from build123d import *

# Parameters (mm, degrees)
BOSS_EXTRU_2_DEPTH      = 50
ESQUISSE5_R             = 1.75
ENL_V_MAT_EXTRU_2_DEPTH = 117.711988712
ESQUISSE6_R             = 1.75
ENL_V_MAT_EXTRU_3_DEPTH = 117.711988712
ENL_V_MAT_EXTRU_5_DEPTH = 44
ESQUISSE8_R             = 5
BOSS_EXTRU_3_DEPTH      = 100
ENL_V_MAT_EXTRU_6_DEPTH = 124.636564171
CONG_1_R                = 2.5
R_VOLUTION1_ANGLE       = 180
BOSS_EXTRU_4_DEPTH      = 1
CONG_2_R                = 10


with BuildPart() as part:
    # Esquisse4 → Boss.-Extru.2 (new body)
    with BuildSketch(Plane.XY):
        Polygon((-14.142135624, 45), (14.142135624, 45), (45, 14.142135624), (45, -14.142135624), (14.142135624, -45), (-14.142135624, -45), (-45, -14.142135624), (-45, 14.142135624), align=None)
    extrude(amount=BOSS_EXTRU_2_DEPTH)

    # Esquisse5 → Enlèv. mat.-Extru.2 (cut, through all)
    with BuildSketch(Plane(origin=(29.571067812, 29.571067812, 0), x_dir=(0, 0, -1), z_dir=(0.7071067811865474, 0.7071067811865477, 0))):
        with Locations(Location((-13.335, 11.665, 0), (0, 0, 90))):
            Circle(ESQUISSE5_R)
        with Locations(Location((-36.665, 11.665, 0), (0, 0, 90))):
            Circle(ESQUISSE5_R)
        with Locations(Location((-13.335, -11.665, 0), (0, 0, 90))):
            Circle(ESQUISSE5_R)
        with Locations(Location((-36.665, -11.665, 0), (0, 0, 90))):
            Circle(ESQUISSE5_R)
    extrude(amount=-ENL_V_MAT_EXTRU_2_DEPTH, mode=Mode.SUBTRACT)

    # Esquisse6 → Enlèv. mat.-Extru.3 (cut, through all)
    with BuildSketch(Plane(origin=(29.571067812, -29.571067812, 0), x_dir=(0, 0, -1), z_dir=(0.7071067811865476, -0.7071067811865476, 0))):
        with Locations(Location((-13.335, 11.665, 0), (0, 0, 90))):
            Circle(ESQUISSE6_R)
        with Locations((-36.665, 11.665)):
            Circle(ESQUISSE6_R)
        with Locations((-13.335, -11.665)):
            Circle(ESQUISSE6_R)
        with Locations((-36.665, -11.665)):
            Circle(ESQUISSE6_R)
    extrude(amount=-ENL_V_MAT_EXTRU_3_DEPTH, mode=Mode.SUBTRACT)

    # Esquisse7 → Enlèv. mat.-Extru.5 (cut)
    with BuildSketch(Plane.XY.offset(50)):
        Polygon((-40, 12.071067812), (-12.071067812, 40), (12.071067812, 40), (40, 12.071067812), (40, -12.071067812), (12.071067812, -40), (-12.071067812, -40), (-40, -12.071067812), align=None)
    extrude(amount=-ENL_V_MAT_EXTRU_5_DEPTH, mode=Mode.SUBTRACT)

    # Esquisse8 → Boss.-Extru.3 (add)
    with BuildSketch(Plane(origin=(0, 0, 0), x_dir=(-1, 0, 0), z_dir=(0, 0, -1))):
        Circle(ESQUISSE8_R)
    extrude(amount=BOSS_EXTRU_3_DEPTH)

    # Esquisse9 → Enlèv. mat.-Extru.6 (cut, through all)
    with BuildSketch(Plane.XY.offset(6)):
        Polygon((-13.017766953, 13.017766953), (-0.289844892, 25.745689014), (-9.128679656, 34.584523779), (-34.584523779, 9.128679656), (-25.745689014, 0.289844892), align=None)
        Polygon((25.745689014, -0.289844892), (34.584523779, -9.128679656), (9.128679656, -34.584523779), (0.289844892, -25.745689014), (13.017766953, -13.017766953), align=None)
        Polygon((-13.017766953, -13.017766953), (-23.624368671, -2.411165235), (-32.463203436, -11.25), (-11.25, -32.463203436), (-2.411165235, -23.624368671), align=None)
        Polygon((2.411165235, 23.624368671), (11.25, 32.463203436), (32.463203436, 11.25), (23.624368671, 2.411165235), (13.017766953, 13.017766953), align=None)
    extrude(amount=-ENL_V_MAT_EXTRU_6_DEPTH, mode=Mode.SUBTRACT)

    # Congé1
    cong_1_edges = [part.edges().sort_by_distance(p)[0] for p in [
        (2.411165235, 23.624368671, 3),
        (11.25, 32.463203436, 3),
        (32.463203436, 11.25, 3),
        (23.624368671, 2.411165235, 3),
        (-2.411165235, -23.624368671, 3),
        (-11.25, -32.463203436, 3),
        (-32.463203436, -11.25, 3),
        (-23.624368671, -2.411165235, 3),
        (25.745689014, -0.289844892, 3),
        (34.584523779, -9.128679656, 3),
        (9.128679656, -34.584523779, 3),
        (0.289844892, -25.745689014, 3),
        (-25.745689014, 0.289844892, 3),
        (-34.584523779, 9.128679656, 3),
        (-9.128679656, 34.584523779, 3),
        (-0.289844892, 25.745689014, 3),
    ]]
    fillet(cong_1_edges, radius=CONG_1_R)

    # Esquisse12 → Révolution1 (revolve)
    with BuildSketch(Plane(origin=(0, 0, -100), x_dir=(-1, 0, 0), z_dir=(0, 0, -1))):
        with BuildLine():
            Line((-5, 0), (5, 0))
            ThreePointArc((5, 0), (0, 5), (-5, 0))
        make_face()
    revolve(axis=Axis((5, 0, -100), (-1, 0, 0)), revolution_arc=R_VOLUTION1_ANGLE)

    # Esquisse13 → Boss.-Extru.4 (add)
    with BuildSketch(Plane.XY.offset(50)):
        Polygon((-45, 14.142135624), (-14.142135624, 45), (14.142135624, 45), (45, 14.142135624), (45, -14.142135624), (14.142135624, -45), (-14.142135624, -45), (-45, -14.142135624), align=None)
        Polygon((-40, 12.071067812), (-12.071067812, 40), (12.071067812, 40), (40, 12.071067812), (40, -12.071067812), (12.071067812, -40), (-12.071067812, -40), (-40, -12.071067812), align=None, mode=Mode.SUBTRACT)
    extrude(amount=BOSS_EXTRU_4_DEPTH)

    # Congé2
    cong_2_edges = [part.edges().sort_by_distance(p)[0] for p in [
        (5, 0, 0),
    ]]
    fillet(cong_2_edges, radius=CONG_2_R)


solid = part.part
Verification items for the finished model (mm, model axes). A direction names the side the tool comes from. Coordinates: 2 decimals unless noted, no trailing zeros. Order: outer loops, then holes, each group sorted by start corner. A loop starts at its lowest first (then second) coordinate and runs counter-clockwise, first axis right, second up.
Item 1: Material ranges on L1, parallel to Y at x = -5.5, z = 23.5; L2, parallel to Z at x = -37, y = -1, recorded low to high.
Filled in:
L1: y = -45 to -40, 40 to 45
L2: z = 0 to 6
Item 2: Section check A-A, the plane z = 20.5. Enter the section's corners in (x, y).
Filled in:
outline: (-45, -14.14) - (-14.14, -45) - (14.14, -45) - (45, -14.14) - (45, 14.14) - (14.14, 45) - (-14.14, 45) - (-45, 14.14) - close; hole (-40, -12.07) - (-12.07, -40) - (12.07, -40) - (40, -12.07) - (40, 12.07) - (12.07, 40) - (-12.07, 40) - (-40, 12.07) - close
Item 3: Release check for a two-part mould opening along X. For faces 1 (the face through (6.793, 28.007, 3.042)), 2 (the face through (-45, 0, 25)), 3 (the face through (29.787, -29.355, 25.143)), 4 (the face through (31.428, 11.277, 2.958)) record: +X half, -X half, draft (parallel to the pull), parting line (faces both ways), or undercut.
Filled in:
face 1: undercut
face 2: -X half
face 3: +X half
face 4: undercut
Item 4: Depth check by flat-ended pin: pin 1 (1.5 mm diameter, centred on x = 16.5, z = 10.5, fed in from +Y); pin 2 (3 mm diameter, centred on y = 20, z = 30.5, fed in from -X); pin 3 (3 mm diameter, centred on y = -23.5, z = 16, fed in from -X); pin 4 (8 mm diameter, centred on y = -17.5, z = 8.5, fed in from +X). Enter the tip coordinate at first touch or a pass-through.
Filled in:
pin 1: stops at y = 43.39
pin 2: stops at x = -40.64
pin 3: stops at x = -37.14
pin 4: stops at x = 45
Item 5: Section check B-B, the plane z = -74. Enter the section's corners in (x, y), then the cut area to 3 significant figures.
Filled in:
outline: circle Ø10 at (0, 0)
area: 78.5 mm2
Item 6: Access from +Z, -Z, +X, -X, +Y, -Y to the whole of each face (thin tool, end or side, straight path). Record for faces 5 (the face through (37.2, -18.4, 12.7)), 6 (the face through (0, 40, 28)), 7 (the face through (3.447, 23.597, 2.958)).
Filled in:
face 5: none
face 6: +Z
face 7: +Z, -Z
